Check sheet for the modelled part. Datum: model origin and axes. Units: mm. Face numbers are marked on the shaded views. Round coordinates to 2 decimals unless told otherwise and drop trailing zeros. Write each loop counter-clockwise with the first axis right and the second up, starting at its lowest first coordinate (ties: lowest second). Pieces come first, ordered by that corner, then holes. Notation, with made-up numbers: (25, 35.25) -> (83, 35.25) arc R12 cw to (83, 43.25) -> close; hole circle Ø7 at (71.25, 13). An arc over 180 degrees is marked (long way). Put each result on its own line as item: value. Start each with the question number.
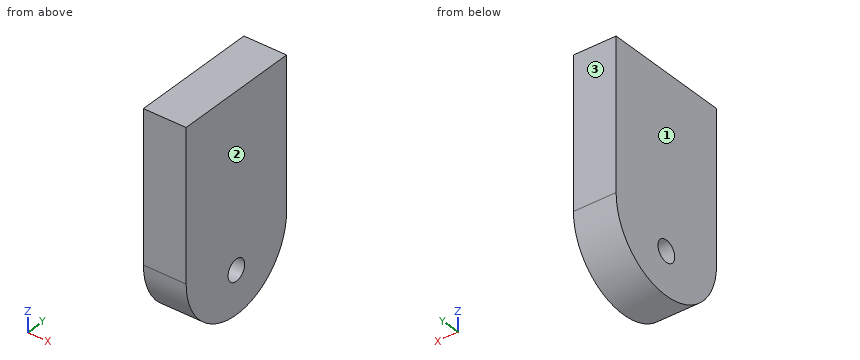
from build123d import *

# Parameters (mm, degrees)
F0_R     = 1.5875
F1_DEPTH = 6.35


with BuildPart() as f1:
    # F0 (on Right) → F1 (new body)
    with BuildSketch(Plane.YZ):
        with BuildLine():
            Line((0, 0), (0, -22.225))
            ThreePointArc((0, -22.225), (9.525, -31.75), (19.05, -22.225))
            Line((19.05, -22.225), (19.05, 0))
            Line((19.05, 0), (0, 0))
        make_face()
        with Locations((9.525, -25.4)):
            Circle(F0_R, mode=Mode.SUBTRACT)
    extrude(amount=F1_DEPTH)


solid = f1.part
1. Material ranges on L1, parallel to Z at x = 3.75, y = 8.25; L2, parallel to Z at x = 6.25, y = 12.75; L3, parallel to Z at x = 4.5, y = 7.25, recorded low to high. Write a range as [from, to].
2. Section check D-D, the plane y = 14. Enter the section's corners in (x, z).
3. Gauge pin test, flat ends, axial feed: P1, Ø10, axis at y = 6.5, z = -8.5, coming from the -X side; P2, Ø2, axis at x = 4.5, y = 15, coming from the -Z side; P3, Ø1.5, axis at x = 1, y = 2, coming from the -Z side. Record the tip position at first contact, or that the pin passes through.
4. Section check B-B, the plane z = -25.4. Enter the section's corners in (x, y), then the cut area to 3 significant figures.
5. Section check C-C, the plane y = 4.5. Enter the section's corners in (x, z).
6. Draft check along X on the marked faces 1, 2 and 3. Enter one of: released by +X, released by -X, zero draft, split by the parting line, or undercut.
Reply:
1. L1: z = [-31.66, -26.35], [-24.45, 0]
1. L2: z = [-31.19, 0]
1. L3: z = [-31.47, 0]
2. outline: (0, -30.63) -> (6.35, -30.63) -> (6.35, 0) -> (0, 0) -> close
3. P1: stops at x = 0
3. P2: stops at z = -30.63
3. P3: stops at z = -28.92
4. outline: (0, 0.54) -> (6.35, 0.54) -> (6.35, 7.94) -> (0, 7.94) -> close; (0, 11.11) -> (6.35, 11.11) -> (6.35, 18.51) -> (0, 18.51) -> close
4. area: 93.9 mm2
5. outline: (0, -30.32) -> (6.35, -30.32) -> (6.35, 0) -> (0, 0) -> close
6. face 1: released by -X
6. face 2: released by +X
6. face 3: zero draft
